from build123d import *

# Parameters (mm, degrees)
SKETCH_2_R          = 12.1
EXTRUDE_1_DEPTH     = 19.05
EXTRUDE_START       = 19.05
SKETCH_2_3_R        = 12.4
SKETCH_2_3_R_2      = 12.1
SKETCH_2_3_R_3      = 3.5
SKETCH_2_3_R_4      = 1.5
EXTRUDE_2_DEPTH     = 18.75
EXTRUDE_START_2     = 37.8
SKETCH_2_4_R        = 3.5
SKETCH_2_4_R_2      = 1.5
EXTRUDE_3_DEPTH     = 2.7
EXTRUDE_START_3     = 40.5
SKETCH_2_5_R        = 1.5
EXTRUDE_4_DEPTH     = 11
SKETCH_4_R          = 1.6
CUT_EXTRUDE_1_DEPTH = 7
SKETCH_5_W          = 5.123568468
SKETCH_5_H          = 1
CUT_EXTRUDE_2_DEPTH = 8
SKETCH_6_R          = 7
SKETCH_6_W          = 5
SKETCH_6_H          = 14
EXTRUDE_5_DEPTH     = 6.7


with BuildPart() as part:
    # 草图2 → 凸台-拉伸1 (new body)
    with BuildSketch(Plane(origin=(0, 0, 0), x_dir=(1, 0, 0), z_dir=(0, 1, 0))):
        with Locations(Location((0, 0, 0), (0, 0, 90))):
            Circle(SKETCH_2_R)
    extrude(amount=EXTRUDE_1_DEPTH)

    # 草图2<3> → 凸台-拉伸2 (add)
    # profile 1 of 4: a face of its own
    with BuildSketch(Plane(origin=(0, 0, 0), x_dir=(1, 0, 0), z_dir=(0, 1, 0)).offset(EXTRUDE_START)):
        with Locations(Location((0, 0, 0), (0, 0, 270))):
            Circle(SKETCH_2_3_R)
        with Locations(Location((0, 0, 0), (0, 0, 90))):
            Circle(SKETCH_2_3_R_2, mode=Mode.SUBTRACT)
    # profile 2 of 4: a face of its own
    with BuildSketch(Plane(origin=(0, 0, 0), x_dir=(1, 0, 0), z_dir=(0, 1, 0)).offset(EXTRUDE_START)):
        with Locations(Location((0, 0, 0), (0, 0, 90))):
            Circle(SKETCH_2_3_R_2)
        Circle(SKETCH_2_3_R_3, mode=Mode.SUBTRACT)
    # profile 3 of 4: a face of its own
    with BuildSketch(Plane(origin=(0, 0, 0), x_dir=(1, 0, 0), z_dir=(0, 1, 0)).offset(EXTRUDE_START)):
        Circle(SKETCH_2_3_R_3)
        Circle(SKETCH_2_3_R_4, mode=Mode.SUBTRACT)
    # profile 4 of 4: a face of its own
    with BuildSketch(Plane(origin=(0, 0, 0), x_dir=(1, 0, 0), z_dir=(0, 1, 0)).offset(EXTRUDE_START)):
        Circle(SKETCH_2_3_R_4)
    extrude(amount=EXTRUDE_2_DEPTH)

    # 草图2<4> → 凸台-拉伸3 (add)
    # profile 1 of 2: a face of its own
    with BuildSketch(Plane(origin=(0, 0, 0), x_dir=(1, 0, 0), z_dir=(0, 1, 0)).offset(EXTRUDE_START_2)):
        with Locations(Location((0, 0, 0), (0, 0, 90))):
            Circle(SKETCH_2_4_R)
        Circle(SKETCH_2_4_R_2, mode=Mode.SUBTRACT)
    # profile 2 of 2: a face of its own
    with BuildSketch(Plane(origin=(0, 0, 0), x_dir=(1, 0, 0), z_dir=(0, 1, 0)).offset(EXTRUDE_START_2)):
        Circle(SKETCH_2_4_R_2)
    extrude(amount=EXTRUDE_3_DEPTH)

    # 草图2<5> → 凸台-拉伸4 (add)
    with BuildSketch(Plane(origin=(0, 0, 0), x_dir=(1, 0, 0), z_dir=(0, 1, 0)).offset(EXTRUDE_START_3)):
        with Locations(Location((0, 0, 0), (0, 0, 270))):
            Circle(SKETCH_2_5_R)
    extrude(amount=EXTRUDE_4_DEPTH)

    # 草图4 → 切除-拉伸1 (cut)
    with BuildSketch(Plane(origin=(0, 37.8, 0), x_dir=(1, 0, 0), z_dir=(0, 1, 0))):
        with Locations(Location((0, 8.5, 0), (0, 0, 270))):
            Circle(SKETCH_4_R)
        with Locations(Location((8.5, 0, 0), (0, 0, 270))):
            Circle(SKETCH_4_R)
        with Locations(Location((0, -8.5, 0), (0, 0, 270))):
            Circle(SKETCH_4_R)
        with Locations(Location((-8.5, 0, 0), (0, 0, 270))):
            Circle(SKETCH_4_R)
    extrude(amount=-CUT_EXTRUDE_1_DEPTH, mode=Mode.SUBTRACT)

    # 草图5 → 切除-拉伸2 (cut)
    with BuildSketch(Plane(origin=(0, 51.5, 0), x_dir=(1, 0, 0), z_dir=(0, 1, 0))):
        with Locations((0, 1.5)):
            Rectangle(SKETCH_5_W, SKETCH_5_H)
    extrude(amount=-CUT_EXTRUDE_2_DEPTH, mode=Mode.SUBTRACT)

    # 草图6 → 凸台-拉伸5 (add)
    with BuildSketch(Plane.XZ):
        with Locations(Location((0, 0, 0), (0, 0, 270))):
            Circle(SKETCH_6_R)
        with Locations((-11.5, 0)):
            Rectangle(SKETCH_6_W, SKETCH_6_H)
    extrude(amount=EXTRUDE_5_DEPTH)


solid = part.part
Read the model definition and answer for the solid it produces. Units are mm, in the model's axes. A direction names the side the tool comes from. Give positions to 0.01 mm unless a question says otherwise; leave off trailing zeros. Loops run counter-clockwise (first coordinate to the right, second up) from the corner with the lowest first, then second, coordinate; pieces in that order, holes last. Notation, with made-up numbers: (-9, 77.25) -> (30, 77.25) arc R10 ccw to (30, 90.25) -> close; hole circle Ø5 at (14, 3.25). An arc over 180 degrees is marked (long way). Answer as CSV lines item,"result".
Item 1: Each of these flat-tipped pins is pushed along its axis until it touches: pin 1 (4 mm diameter, centred on y = -1, z = 5, fed in from +X); pin 2 (5 mm diameter, centred on x = 4, y = 0.5, fed in from -Z); pin 3 (1.5 mm diameter, centred on x = -12, y = -5, fed in from +Z). Where does it stop, or does it pass through?
Returned:
pin 1,"stops at x = 11.65"
pin 2,"stops at z = -12.01"
pin 3,"stops at z = 7"
Item 2: For faces 4 (the face through (0.45, 45.92, 1.43)), 5 (the face through (-6.834, -3.303, 1.517)), 6 (the face through (-12, -3, 7)), determine the directions among +Z, -Z, +X, -X, +Y, -Y from which every point of the face is accessible in a straight line to the end or side of a thin tool.
Returned:
face 4,"+Y"
face 5,"-Y"
face 6,"+Z, +X, -X, -Y"
Item 3: Find section D-D on z = 8.75. Give the vertices of the cut face in (x, y).
Returned:
outline,"(-8.79, 19.05) -> (-8.36, 19.05) -> (-8.36, 0) -> (8.36, 0) -> (8.36, 19.05) -> (8.79, 19.05) -> (8.79, 37.8) -> (1.58, 37.8) -> (1.58, 30.8) -> (-1.58, 30.8) -> (-1.58, 37.8) -> (-8.79, 37.8) -> close"
Item 4: Find section C-C on y = 21. Give the vertices of the cut face in (x, z).
Returned:
outline,"circle Ø24.8 at (0, 0)"
Item 5: Consider line 1 (X direction, y = 32, z = 0); line 2 (Y direction, x = -2.5, z = 10.75); line 3 (Y direction, x = -11, z = 3.75). Determine where each line is inside the solid, lowest interval first. Write a range as [from, to].
Returned:
line 1,"x = [-12.4, -10.1], [-6.9, 6.9], [10.1, 12.4]"
line 2,"y = [0, 37.8]"
line 3,"y = [-6.7, 37.8]"
Item 6: Determine the mould class of faces 1 (the face through (-12, -6.7, 0)), 2 (the face through (3.417, 39.131, 0.759)), 3 (the face through (9, 30.8, 0)) for opening direction X: +X half, -X half, draft (parallel to the pull), parting line (faces both ways), or undercut.
Returned:
face 1,"draft"
face 2,"parting line"
face 3,"undercut"
